from build123d import *

# Parameters (mm, degrees)
SALIENTE_EXTRUIR1_START = -5
CROQUIS3_R              = 3.650933922
SALIENTE_EXTRUIR1_DEPTH = 5
REDONDEO1_R             = 0.5
CHAFL_N1_SIZE           = 0.1


with BuildPart() as part:
    # Croquis1 → Revolución1 (revolve)
    with BuildSketch(Plane.XY, mode=Mode.PRIVATE) as revoluci_n1_sk:
        Polygon((0.2, 0), (0.2, 1.2), (1.6, 3.199407209), (1.6, 15), (3, 15), (3, 9.5), (3.650933922, 9.5), (3.650933922, 4.5), (0.5, 0), align=None)
    revolve(revoluci_n1_sk.sketch.rotate(Axis((0, 0, 0), (0, 1, 0)), 90), axis=Axis((0, 0, 0), (0, 1, 0)))

    # Croquis3 → Saliente-Extruir1 (add)
    with BuildSketch(Plane(origin=(0, 9.5, 0), x_dir=(1, 0, 0), z_dir=(0, 1, 0)).offset(SALIENTE_EXTRUIR1_START)):
        Polygon((-2.309401077, -4), (2.309401077, -4), (4.618802154, 0), (2.309401077, 4), (-2.309401077, 4), (-4.618802154, 0), align=None)
        Circle(CROQUIS3_R, mode=Mode.SUBTRACT)
    extrude(amount=SALIENTE_EXTRUIR1_DEPTH)

    # Redondeo1
    redondeo1_edges = [part.edges().sort_by_distance(p)[0] for p in [
        (0, 0, 0.5),
    ]]
    fillet(redondeo1_edges, radius=REDONDEO1_R)

    # Chaflán1
    chafl_n1_edges = [part.edges().sort_by_distance(p)[0] for p in [
        (0, 15, 1.6),
    ]]
    chamfer(chafl_n1_edges, length=CHAFL_N1_SIZE)

    # Croquis5 → Cortar-Revolución1 (revolve, cut)
    with BuildSketch(Plane.XY, mode=Mode.PRIVATE) as cortar_revoluci_n1_sk:
        Polygon((3.650933922, 4.5), (4.618802154, 5.882259086), (4.618802154, 4.5), align=None)
    revolve(cortar_revoluci_n1_sk.sketch.rotate(Axis((0, 15, 0), (0, -1, 0)), 90), axis=Axis((0, 15, 0), (0, -1, 0)), mode=Mode.SUBTRACT)


solid = part.part
For this review, take the finished solid that the model builds, in its own axes (mm). A direction names the side the tool comes from. Give positions to 0.01 mm unless a question says otherwise; leave off trailing zeros. Loops run counter-clockwise (first coordinate to the right, second up) from the corner with the lowest first, then second, coordinate; pieces in that order, holes last. Notation, with made-up numbers: M 56,83.25 L 88,83.25 A23 cw 88,106.25 Z; hole C 13,32 d7. An arc over 180 degrees is marked long. Answer as a JSON object with one key per item and string values. Group by question number.
Q1. Mouldability with a two-part tool opening along X and no side actions: class faces 3 (the cylindrical face through (-0.481, 9.132, -1.526)), 4 (the flat face through (3.448, 7.218, 2.028)), 5 (the conical face through (0.584, 1.769, 0.13)), 6 (the flat face through (0, 7, 4)) as +X half, -X half, draft (parallel to the pull), parting line (faces both ways), or undercut.
Q2. Tool access review of faces 1 (the flat face through (-3.48, 7.22, 1.97)), 2 (the cylindrical face through (-0.9, 12.21, -2.86)): name each direction out of +Z, -Z, +X, -X, +Y, -Y from which nothing blocks a thin tool from reaching the whole face with its end or side.
Q3. Insertion check: P1, Ø1.5, axis at x = 2, z = -1.5, coming from the -Y side; P2, Ø1, axis at x = 3.5, y = 8.5, coming from the +Z side; P3, Ø4, axis at y = 10.5, z = -2, coming from the +X side. Each pin has a flat end and moves straight along its axis. Give the tip position at first contact, or say it passes through.
Q4. For probe 1 along X at (y, z) = (4.75, -1.25); probe 2 along X at (y, z) = (6, 0.25); probe 3 along Y at (x, z) = (1.25, 0.75), list the stretches that pass through material, from the lowest coordinate up. Write a range as [from, to].
Q5. Add section C-C on y = 4.75. Give the boundary of the cut face in (x, z).
Q6. Add section B-B on y = 12.5. Give the boundary of the cut face in (x, z), and give its area (3 significant figures).
Q7. Add section A-A on y = 6.25. Give the boundary of the cut face in (x, z).
Checked values:
{
 "1": {"face 3": "undercut", "face 4": "+X half", "face 5": "undercut", "face 6": "draft"},
 "2": {"face 1": "+Z, -X, +Y, -Y", "face 2": "+Y"},
 "3": {"P1": "y = 1.79", "P2": "z = 2.8", "P3": "x = 4.46"},
 "4": {"probe 1": "[-3.62, -1], [1, 3.62]", "probe 2": "[-4.47, -1.58], [1.58, 4.47]", "probe 3": "[1.37, 3]"},
 "5": {"outline": "C 0,0 d7.65; hole C 0,0 d3.2"},
 "6": {"outline": "C 0,0 d6; hole C 0,0 d3.2", "area": "20.2 mm²"},
 "7": {"outline": "M -4.62,0 L -2.31,-4 L 2.31,-4 L 4.62,0 L 2.31,4 L -2.31,4 Z; hole C 0,0 d3.2"}
}
